Could you check a few things on this model? Use its own coordinates, in mm. A direction names the side the tool comes from. Round coordinates to 2 decimals unless told otherwise and drop trailing zeros. Loops run counter-clockwise (first coordinate to the right, second up) from the corner with the lowest first, then second, coordinate; pieces in that order, holes last. Notation, with made-up numbers: (14, -18) - (70, -18) arc R12 cw to (70, 0) - close; hole circle Ø2 at (73, -1.75). An arc over 180 degrees is marked (long way). Use one line per item in the form item = value.
```python
from build123d import *

# Parameters (mm, degrees)
BOSS_EXTRUDE1_DEPTH = 184.15
SKETCH2_R           = 3.175
CUT_EXTRUDE1_DEPTH  = 381


with BuildPart() as part:
    # Sketch1 → Boss-Extrude1 (new body, symmetric)
    with BuildSketch(Plane.XY):
        with BuildLine():
            Line((0, -133.35), (0, -130.175))
            ThreePointArc((0, -130.175), (92.047625241, -92.047625241), (130.175, 0))
            Line((130.175, 0), (130.175, 25.4))
            Line((130.175, 25.4), (133.35, 25.4))
            Line((133.35, 25.4), (133.35, 0))
            ThreePointArc((133.35, 0), (94.292689271, -94.292689271), (0, -133.35))
        make_face()
    extrude(amount=BOSS_EXTRUDE1_DEPTH, both=True)

    # Sketch2 → Cut-Extrude1 (cut)
    with BuildSketch(Plane(origin=(133.35, 0, 0), x_dir=(0, 0, -1), z_dir=(1, 0, 0))):
        with Locations((0, 12.7)):
            Circle(SKETCH2_R)
        with Locations((85.725, 12.7)):
            Circle(SKETCH2_R)
        with Locations((-85.725, 12.7)):
            Circle(SKETCH2_R)
        with Locations((-171.45, 12.7)):
            Circle(SKETCH2_R)
        with Locations((171.45, 12.7)):
            Circle(SKETCH2_R)
    extrude(amount=-CUT_EXTRUDE1_DEPTH, mode=Mode.SUBTRACT)


solid = part.part
```
1. On a 3-axis mill with a long thin cutter (end or side, diameter ignored), from which of +Z, -Z, +X, -X, +Y, -Y can I reach the whole of each face in a straight line? I mean faces 1 (the face through (130.175, 10, 3)), 2 (the face through (133.35, 16, 3)). Say none if no direction works.
Solution:
face_1 = +Z, -Z, -X, +Y
face_2 = +Z, -Z, +X, +Y, -Y
2. If we section it at C-C, the plane y = -34: Write out the boundary of the cut face in (x, z).
Solution:
outline = (125.66, -184.15) - (128.94, -184.15) - (128.94, 184.15) - (125.66, 184.15) - close
3. For P1, Ø6, axis at x = 74, z = 11.5, coming from the -Y side; P2, Ø8.5, axis at y = 12.7, z = -85.725, coming from the +X side; P3, Ø8.5, axis at y = 12.7, z = 85.725, coming from the -X side (3 decimals); P4, Ø6, axis at x = 106, z = -16.5, coming from the +Y side, each with a flat end and sliding along its axis, tell me the tip position at first contact or that it passes through.
Solution:
P1 = -112.88
P2 = 133.35
P3 = 130.175
P4 = -71.17
4. If we section it at A-A, the plane z = 60: Write out the boundary of the cut face in (x, y) (3 decimals), plus the area to 3 significant figures.
Solution:
outline = (0, -133.35) arc R133.35 ccw to (133.35, 0) - (133.35, 25.4) - (130.175, 25.4) - (130.175, 0) arc R130.175 cw to (0, -130.175) - close
area = 738 mm^2
5. Please list where these lines run through material, in increasing order: line 1 along Z through (x, y) = (131, 12); line 2 along X through (y, z) = (-3, 84); line 3 along X through (y, z) = (9.5, -58) (3 decimals).
Solution:
line_1 = -184.15 to -174.55, -168.35 to -88.82, -82.63 to -3.1, 3.1 to 82.63, 88.82 to 168.35, 174.55 to 184.15
line_2 = 130.14 to 133.32
line_3 = 130.175 to 133.35
6. We'd pull the mould along Z, two halves only. Please class faces 3 (the face through (106, -77, -184.15)), 4 (the face through (91.03, -93.054, 2.578)), 5 (the face through (131.78, 12.84, -168.28)): +Z half, -Z half, draft (parallel to the pull), parting line (faces both ways), or undercut.
Solution:
face_3 = -Z half
face_4 = draft
face_5 = undercut
7. If we section it at B-B, the plane x = 49: Write out the boundary of the cut face in (y, z), plus the area to 3 significant figures.
Solution:
outline = (-124.02, -184.15) - (-120.6, -184.15) - (-120.6, 184.15) - (-124.02, 184.15) - close
area = 1,260 mm^2
